Build history of the part. All positions in model axes, mm. Face numbers are marked on the shaded views. A direction names the side the tool comes from. Round coordinates to 2 decimals unless told otherwise and drop trailing zeros. Loops run counter-clockwise (first coordinate to the right, second up) from the corner with the lowest first, then second, coordinate; pieces in that order, holes last.
from build123d import *

# Parameters (mm, degrees)
BOSS_EXTRUDE1_DEPTH       = 6.35
FILLET1_R                 = 6.35
F_1_4_CLEARANCE_HOLE1_D   = 6.7564
TAP_DRILL_FOR_6_32_TAP1_D = 2.7051


with BuildPart() as part:
    # Sketch1 → Boss-Extrude1 (new body)
    with BuildSketch(Plane(origin=(0, 0, 0), x_dir=(1, 0, 0), z_dir=(0, 1, 0))):
        with BuildLine():
            Line((0, 0), (114.3, 0))
            Line((114.3, 0), (114.3, 15.075180871))
            Line((114.3, 15.075180871), (113.175058985, 15.632165638))
            ThreePointArc((113.175058985, 15.632165638), (76.8604, 24.13), (113.175058985, 32.627834362))
            Line((113.175058985, 32.627834362), (114.3, 33.184819129))
            Line((114.3, 33.184819129), (114.3, 48.26))
            Line((114.3, 48.26), (0, 48.26))
            Line((0, 48.26), (0, 0))
        make_face()
        with BuildLine():
            Line((35.56, 41.783), (48.26, 41.783))
            ThreePointArc((48.26, 41.783), (65.913, 24.13), (48.26, 6.477))
            Line((48.26, 6.477), (35.56, 6.477))
            ThreePointArc((35.56, 6.477), (17.907, 24.13), (35.56, 41.783))
        make_face(mode=Mode.SUBTRACT)
    extrude(amount=BOSS_EXTRUDE1_DEPTH)

    # Fillet1
    fillet1_edges = [part.edges().sort_by_distance(p)[0] for p in [
        (0, 3.175, 0),
        (0, 3.175, -48.26),
        (114.3, 3.175, -48.26),
        (114.3, 3.175, 0),
    ]]
    fillet(fillet1_edges, radius=FILLET1_R)

    # 1/4 Clearance Hole1 (through all)
    with Locations(Plane(origin=(0, 6.35, 0), x_dir=(1, 0, 0), z_dir=(0, 1, 0))):
        with Locations((7.9375, 40.005), (7.9375, 8.255)):
            Hole(F_1_4_CLEARANCE_HOLE1_D / 2)

    # Tap Drill for #6-32 Tap1 (through all)
    with Locations(Plane(origin=(0, 6.35, 0), x_dir=(1, 0, 0), z_dir=(0, 1, 0))):
        with Locations((82.042, 43.18), (109.982, 43.18), (109.982, 5.08), (82.042, 5.08), (96.012, 24.13)):
            Hole(TAP_DRILL_FOR_6_32_TAP1_D / 2)


solid = part.part
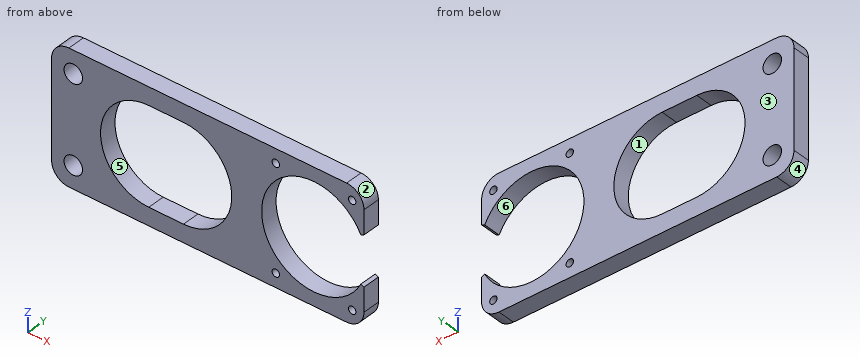
(1) Which spindle directions (+Z, -Z, +X, -X, +Y, -Y) get a long thin tool onto all of the face, cutting with end or side? Do the marked faces 1 and 2. Say none if no direction does.
Responses:
face 1: +Y, -Y
face 2: +Z, +X, +Y, -Y
(2) Slice it at A-A on z = -24.13. List the corners of the cut face in (x, y).
Responses:
outline: (0, 0) - (17.91, 0) - (17.91, 6.35) - (0, 6.35) - close; (65.91, 0) - (76.86, 0) - (76.86, 6.35) - (65.91, 6.35) - close
(3) Probe line 1 (Z direction, x = 8, y = 3.25); line 2 (Z direction, x = 39.5, y = 3); line 3 (X direction, y = 3.5, z = -24.13). List the from-to ranges inside material, lowest first.
Responses:
line 1: z = -48.26 to -43.38, -36.63 to -11.63, -4.88 to 0
line 2: z = -48.26 to -41.78, -6.48 to 0
line 3: x = 0 to 17.91, 65.91 to 76.86
(4) Slice it at D-D on z = -2.5. List the corners of the cut face in (x, y).
Responses:
outline: (1.3, 0) - (113, 0) - (113, 6.35) - (1.3, 6.35) - close
(5) Slice it at C-C on y = 1. Count the separate pieces of the cut face and the enclosed holes in it, plus the area to 3 significant figures.
Responses:
separate pieces: 1
enclosed holes: 7
area: 2,810 mm2
(6) Slice it at B-B on x = 43.5. List the corners of the cut face in (y, z).
Responses:
outline: (0, -48.26) - (6.35, -48.26) - (6.35, -41.78) - (0, -41.78) - close; (0, -6.48) - (6.35, -6.48) - (6.35, 0) - (0, 0) - close
(7) Pull direction X, two halves, no side cores. Call the marked faces 3, 4, 5 and 6: +X half, -X half, draft (parallel to the pull), parting line (faces both ways), or undercut.
Responses:
face 3: draft
face 4: -X half
face 5: undercut
face 6: undercut
